from build123d import *

# Parameters (mm, degrees)
F0_W       = 76.2
F0_H       = 76.2
F0_W_2     = 73.152
F0_H_2     = 73.152
F1_DEPTH   = 1092.2
F6_D       = 15.875
F6_ON_F5_D = 15.875
F8_DEPTH   = 1.524
F9_DEPTH   = 1.524
F10_W      = 76.2
F10_H      = 353.2152473927
F10_R      = 7.9375
F11_DEPTH  = 3.048


with BuildPart() as f1:
    # F0 (on Right) → F1 (new body)
    with BuildSketch(Plane.YZ):
        Rectangle(F0_W, F0_H)
        Rectangle(F0_W_2, F0_H_2, mode=Mode.SUBTRACT)
    extrude(amount=F1_DEPTH)

    # F6 (through all)
    with Locations(Plane.XZ.offset(76.2)):
        with Locations((38.1, 0), (88.9, 0), (139.7, 0), (190.5, 0), (241.3, 0), (292.1, 0), (342.9, 0), (393.7, 0), (444.5, 0), (495.3, 0), (546.1, 0), (596.9, 0), (647.7, 0), (698.5, 0), (749.3, 0), (800.1, 0), (850.9, 0), (901.7, 0), (952.5, 0), (1003.3, 0)):
            Hole(F6_D / 2)

    # F6 on F5 (through all)
    with Locations(Plane.XY.offset(76.2)):
        with Locations((317.5, 0), (469.9, 0), (622.3, 0), (774.7, 0), (927.1, 0)):
            Hole(F6_ON_F5_D / 2)

    # F7 (on Front) → F8 (join)
    with BuildSketch(Plane.XZ):
        with BuildLine():
            Line((228.6, -38.1), (0, -38.1))
            Line((0, -38.1), (0, -63.9625564218))
            ThreePointArc((0, -63.9625564218), (33.2066453993, -97.1692018211), (0, -130.3758472204))
            Line((0, -130.3758472204), (0, -190.5))
            Line((0, -190.5), (23.9939857274, -190.5))
            Line((23.9939857274, -190.5), (228.6, -54.1826970875))
            Line((228.6, -54.1826970875), (228.6, -38.1))
        make_face()
    extrude(amount=F8_DEPTH)

    # F7 (on Front) → F9 (join)
    with BuildSketch(Plane.XZ):
        with BuildLine():
            Line((228.6, -38.1), (0, -38.1))
            Line((0, -38.1), (0, -63.9625564218))
            ThreePointArc((0, -63.9625564218), (33.2066453993, -97.1692018211), (0, -130.3758472204))
            Line((0, -130.3758472204), (0, -190.5))
            Line((0, -190.5), (23.9939857274, -190.5))
            Line((23.9939857274, -190.5), (228.6, -54.1826970875))
            Line((228.6, -54.1826970875), (228.6, -38.1))
        make_face()
    extrude(amount=-F9_DEPTH)

    # F10 (on Right) → F11 (join)
    with BuildSketch(Plane.YZ):
        with Locations((0, -100.8058041334)):
            Rectangle(F10_W, F10_H)
        with Locations((0, -252.0134278297)):
            Circle(F10_R, mode=Mode.SUBTRACT)
        with Locations((0, -99.6134278297)):
            Circle(F10_R, mode=Mode.SUBTRACT)
        with Locations((0, 52.7865721703)):
            Circle(F10_R, mode=Mode.SUBTRACT)
    extrude(amount=F11_DEPTH)

    # F13: F1 across plane


with BuildPart() as f1_1:
    add(f1.part)
    add(f1.part.mirror(Plane.YZ.offset(546.1)))


solid = f1_1.part
Verification items for the finished model (mm, model axes). A direction names the side the tool comes from. Coordinates: 2 decimals unless noted, no trailing zeros. Write each loop counter-clockwise with the first axis right and the second up, starting at its lowest first coordinate (ties: lowest second). Pieces come first, ordered by that corner, then holes. Notation, with made-up numbers: M 47.25,-14.75 L 58.25,-14.75 A19 ccw 58.25,1.25 Z; hole C -25,54.25 d8. An arc over 180 degrees is marked long. One line per question, with ' | ' between items.
1) Material ranges on L1, parallel to X at y = 31, z = -185.5; L2, parallel to Y at x = 662.5, z = -21.5, recorded low to high.
Solutions:
L1: 0 to 3.05, 1089.15 to 1092.2 | L2: -38.1 to -36.58, 36.58 to 38.1
2) Release check for a two-part mould opening along Z. For faces 6 (the face through (967.34, -0.02, -123.3)), 7 (the face through (538, 36.576, -9)), 8 (the face through (538, -1, 36.576)), 9 (the face through (538, -1, 38.1)) record: +Z half, -Z half, draft (parallel to the pull), parting line (faces both ways), or undercut.
Solutions:
face 6: -Z half | face 7: undercut | face 8: undercut | face 9: +Z half
3) Sectioned sample at A-A on z = -213. Record the cut outline in (x, y).
Solutions:
outline: M 0,-38.1 L 3.05,-38.1 L 3.05,38.1 L 0,38.1 Z; M 1089.15,-38.1 L 1092.2,-38.1 L 1092.2,38.1 L 1089.15,38.1 Z
4) Access from +Z, -Z, +X, -X, +Y, -Y to the whole of each face (thin tool, end or side, straight path). Record for faces 1 (the face through (1003, -1.524, -96)), 2 (the face through (3.048, -1, 61)), 3 (the face through (3.048, -1, 1)), 4 (the face through (1003, 1.524, -96)), 5 (the face through (124.86, -0.02, -123.3)).
Solutions:
face 1: -Z, -Y | face 2: +Z, +Y, -Y | face 3: none | face 4: -Z, +Y | face 5: -Z, +Y, -Y
5) Depth check by flat-ended pin: pin 1 Ø1 at (y, z) = (0.5, -55.5) entering from -X; pin 2 Ø5 at (x, y) = (625.5, -30) entering from +Z; pin 3 Ø2 at (x, y) = (417, -21) entering from -Z. Enter the tip coordinate at first touch or a pass-through.
Solutions:
pin 1: x = 0 | pin 2: z = 38.1 | pin 3: z = -38.1
6) Sectioned sample at B-B on x = 720. Record the cut outline in (y, z).
Solutions:
outline: M -38.1,-38.1 L 38.1,-38.1 L 38.1,38.1 L -38.1,38.1 Z; hole M -36.58,-36.58 L 36.58,-36.58 L 36.58,36.58 L -36.58,36.58 Z
